Can you work these out from the model? Positions are in its coordinate system, mm. A direction names the side the tool comes from. Round coordinates to 2 decimals unless told otherwise and drop trailing zeros. Order: outer loops, then holes, each group sorted by start corner. A loop starts at its lowest first (then second) coordinate and runs counter-clockwise, first axis right, second up.
Q1. If we section it at A-A (z = 8): Please give me the cut outline in (x, y).
Q2. If I drill on line 1 (X direction, y = -7.5, z = 36.5); line 2 (Z direction, x = 1, y = 11); line 3 (X direction, y = 15, z = 37), over which ranges is the centre line in solid material (lowest first)?
Q3. If we section it at D-D (y = -29): Please give me the cut outline in (x, z), plus the area to 3 significant figures.
Q4. If we section it at B-B (y = -23): Please give me the cut outline in (x, z).
Q5. Will these pins go through, and if not, where does the flat tip stop? P1, Ø3.5, axis at x = 0, z = 52.5, coming from the +Y side; P2, Ø3, axis at x = 9.5, y = 13.5, coming from the +Z side; P3, Ø10, axis at x = -3, z = 18.5, coming from the -Y side.
Q6. If we section it at C-C (z = 52.5): Please give me the cut outline in (x, y).
Q7. We'd pull the mould along Y, two halves only. Please class faces 4 (the face through (0, 2, 54)), 5 (the face through (11.836, -7.979, 34.69)), 6 (the face through (-0.05, 14.79, 29.88)), 7 (the face through (2.1, 2.4, 44)): pulls with the +Y half, pulls with the -Y half, needs draft (parallel to the pull), parting line crosses it, or undercut.
Q8. For faces 1 (the face through (0, 0, 0)), 2 (the face through (-14.145, -7.979, 34.69)), 3 (the face through (-0.759, -23.03, 4.583)), which set-ups out of +Z, -Z, +X, -X, +Y, -Y let a thin tool reach every point of the face, with its end or its side?
from build123d import *

# Parameters (mm, degrees)
F0_R      = 19.5
F1_DEPTH  = 39
F2_R      = 10
F3_DEPTH  = 5
F4_R      = 3
F5_DEPTH  = 15
F7_D      = 2.5
F7_DEPTH  = 8.5
F7_TIP    = 0.7510757738
F8_W      = 4.472135955
F8_H      = 1
F9_DEPTH  = 10
F10_R     = 3.5
F11_DEPTH = 27
F12_R     = 2.5
F13_DEPTH = 10


with BuildPart() as f1:
    # F0 (on Top) → F1 (new body)
    with BuildSketch(Plane.XY):
        Circle(F0_R)
    extrude(amount=F1_DEPTH)

    # F2 (on face) → F3 (join)
    with BuildSketch(Plane.XY.offset(39)):
        Circle(F2_R)
    extrude(amount=F3_DEPTH)

    # F4 (on face) → F5 (join)
    with BuildSketch(Plane.XY.offset(44)):
        Circle(F4_R)
    extrude(amount=F5_DEPTH)

    # F7
    with Locations(Plane.XY.offset(39)):
        with Locations((0, 15), (-12.9903810568, -7.5), (12.9903810568, -7.5)):
            Hole(F7_D / 2, depth=F7_DEPTH)
            with Locations((0, 0, -(F7_DEPTH + F7_TIP / 2))):  # 118° drill point
                Cone(0, F7_D / 2, F7_TIP, mode=Mode.SUBTRACT)

    # F8 (on face) → F9 (cut)
    with BuildSketch(Plane.XY.offset(59)):
        with Locations((0, 2.5)):
            Rectangle(F8_W, F8_H)
    extrude(amount=-F9_DEPTH, mode=Mode.SUBTRACT)

    # F10 (on Front) → F11 (join)
    with BuildSketch(Plane.XZ):
        with Locations((0, 8)):
            Circle(F10_R)
    extrude(amount=F11_DEPTH)

    # F12 (on face) → F13 (join)
    with BuildSketch(Plane.XZ.offset(27)):
        with Locations((0, 8)):
            Circle(F12_R)
    extrude(amount=F13_DEPTH)


solid = f1.part
Solution:
1. outline: (-3.5, -27) - (-2.5, -27) - (-2.5, -37) - (2.5, -37) - (2.5, -27) - (3.5, -27) - (3.5, -19.18) arc R19.5 ccw (long way) to (-3.5, -19.18) - close
2. line 1: x = -18 to -14.24, -11.74 to 11.74, 14.24 to 18
2. line 2: z = 0 to 39
2. line 3: x = -12.46 to -1.25, 1.25 to 12.46
3. outline: circle Ø5 at (0, 8)
3. area: 19.6 mm2
4. outline: circle Ø7 at (0, 8)
5. P1: stops at y = 2
5. P2: stops at z = 39
5. P3: stops at y = -19.5
6. outline: (-2.24, 2) arc R3 ccw (long way) to (2.24, 2) - close
7. face 4: pulls with the +Y half
7. face 5: undercut
7. face 6: undercut
7. face 7: needs draft
8. face 1: -Z, +X, -X, +Y, -Y
8. face 2: +Z
8. face 3: -Y
